Autodesk Inventor part; units mm, degrees
ref_plane "YZ Plane" through (0, 0, 0) normal (1, 0, 0) x (0, 1, 0)
ref_plane "XZ Plane" through (0, 0, 0) normal (0, 1, 0) x (-1, 0, 0)
ref_plane "XY Plane" through (0, 0, 0) normal (0, 0, 1) x (1, 0, 0)
sketch "Sketch1" plane through (0, 0, 0) normal (0, 1, 0) x (-1, 0, 0)
  circle A0 centre (0, 0) radius 6.25
  circle A1 centre (0, 0) radius 15
  dimension "d0" = 12.5
  dimension "d1" = 30
extrude "Extrusion1" add sketch "Sketch1" along normal blind 7
fillet "Fillet1" radius 1 2 edges at (15, 7, 0) (15, 0, 0)
fillet "Fillet2" radius 1 2 edges at (6.25, 7, 0) (6.25, 0, 0)
properties part number "wheel"
Can you work these out from the model? Positions are in its coordinate system, mm. Round coordinates to 2 decimals unless told otherwise and drop trailing zeros. Loops run counter-clockwise (first coordinate to the right, second up) from the corner with the lowest first, then second, coordinate; pieces in that order, holes last. Notation, with made-up numbers: (80, -14) - (94, -14) arc R15 cw to (94, -9) - close; hole circle Ø1 at (84.5, 83). An arc over 180 degrees is marked (long way). Answer in a Markdown table with one row per item. Add a question column.
Q1. We'd pull the mould along X, two halves only. Please class faces 1 (the cylindrical face through (-5.96, 3.46, -1.88)), 2 (the cylindrical face through (14.985, 3.465, -0.66)), 3 (the flat face through (-6, 7, -6)): pulls with the +X half, pulls with the -X half, needs draft (parallel to the pull), parting line crosses it, or undercut.
Q2. I want a section at C-C on y = 4.25. List the corners of the cut face in (x, z) for me, and give its area (3 significant figures).
Q3. I want a section at A-A on z = 0. List the corners of the cut face in (x, y) for me.
Q4. For pin 1 Ø3 at (x, y) = (8, 1) entering from -Z; pin 2 Ø4 at (x, y) = (-7, 6) entering from -Z; pin 3 Ø4 at (y, z) = (1.5, -5) entering from -X, each with a flat end and sliding along its axis, tell me the tip position at first contact or that it passes through.
Q5. I want a section at B-B on x = 0. List the corners of the cut face in (y, z) for me.
Q6. I need wall thicknesses on L1, parallel to Z at x = 0, y = 5; L2, parallel to X at y = 6.25, z = -0.25; L3, parallel to Z at x = 4.25, y = 4.5. Which ranges of each line are inside material? Lowest first, please.
A:
| question | item | result |
|---|---|---|
| 1 | face 1 | undercut |
| 1 | face 2 | parting line crosses it |
| 1 | face 3 | needs draft |
| 2 | outline | circle Ø30 at (0, 0); hole circle Ø12.5 at (0, 0) |
| 2 | area | 584 mm^2 |
| 3 | outline | (-15, 1) arc R1 ccw to (-14, 0) - (-7.25, 0) arc R1 ccw to (-6.25, 1) - (-6.25, 6) arc R1 ccw to (-7.25, 7) - (-14, 7) arc R1 ccw to (-15, 6) - close; (6.25, 1) arc R1 ccw to (7.25, 0) - (14, 0) arc R1 ccw to (15, 1) - (15, 6) arc R1 ccw to (14, 7) - (7.25, 7) arc R1 ccw to (6.25, 6) - close |
| 4 | pin 1 | z = -13.52 |
| 4 | pin 2 | z = -14.14 |
| 4 | pin 3 | x = -14.7 |
| 5 | outline | (0, -14) arc R1 ccw to (1, -15) - (6, -15) arc R1 ccw to (7, -14) - (7, -7.25) arc R1 ccw to (6, -6.25) - (1, -6.25) arc R1 ccw to (0, -7.25) - close; (0, 7.25) arc R1 ccw to (1, 6.25) - (6, 6.25) arc R1 ccw to (7, 7.25) - (7, 14) arc R1 ccw to (6, 15) - (1, 15) arc R1 ccw to (0, 14) - close |
| 6 | L1 | -15 to -6.25, 6.25 to 15 |
| 6 | L2 | -14.97 to -6.28, 6.28 to 14.97 |
| 6 | L3 | -14.39 to -4.58, 4.58 to 14.39 |
